Drawing for the job (mm, zero at the part's lowest x, y, z). Coordinates: 2 decimals unless noted, no trailing zeros. Write each loop counter-clockwise with the first axis right and the second up, starting at its lowest first coordinate (ties: lowest second). Pieces come first, ordered by that corner, then holes. Notation, with made-up numbers: M 35,-26 L 59,-26 A29 ccw 59,1 Z; hole C 68,64.5 d9. An arc over 180 degrees is marked long. Use a Markdown table: item, result. Add a question column.
Q1. Wall check: L1, parallel to Y at x = 7, z = 17.78 (3 decimals); L2, parallel to Y at x = 4.25, z = 18.5; L3, parallel to Z at x = 7.5, y = 101.6. Give the ranges that are in metal, low to high. Write a range as from..to.
Q2. Pin check, flat tip, straight feed: pin 1 Ø2 at (y, z) = (25.4, 5.92) entering from +X. Stop position of the tip, or through.
Q3. Slice it at C-C on x = 4. Count the separate pieces of the cut face and the enclosed holes in it, then the cut area to 3 significant figures.
Q4. Slice it at A-A on y = 101.6. Write the cut outline in (x, z) (1 decimal), then the cut area to 3 significant figures.
Q5. Slice it at B-B on y = 63.5. Write the cut outline in (x, z) (1 decimal).
Q6. Slice it at D-D on z = 15.75. Write the cut outline in (x, y) (1 decimal).
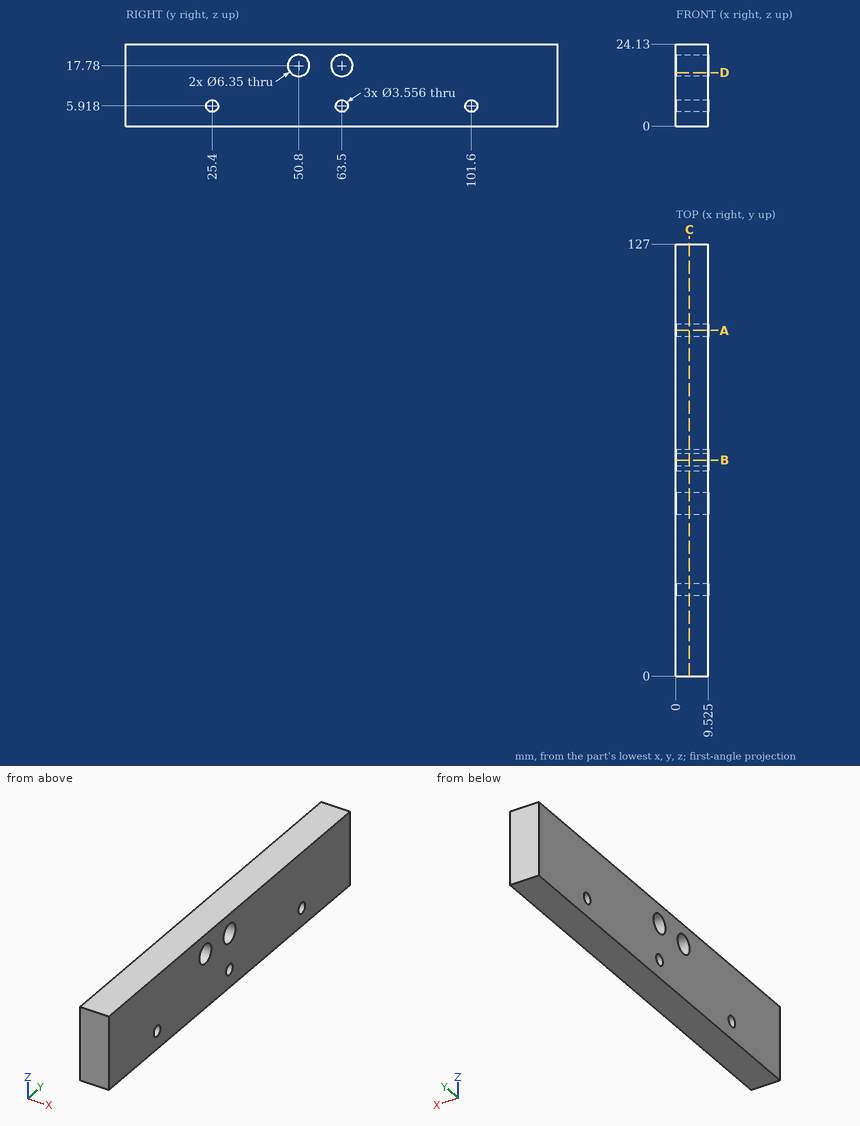
Recorded:
| question | item | result |
|---|---|---|
| 1 | L1 | 0..47.625, 53.975..60.325, 66.675..127 |
| 1 | L2 | 0..47.71, 53.89..60.41, 66.59..127 |
| 1 | L3 | 0..4.14, 7.7..24.13 |
| 2 | pin 1 | through |
| 3 | separate pieces | 1 |
| 3 | enclosed holes | 5 |
| 3 | area | 2,970 mm² |
| 4 | outline | M 0,0 L 9.5,0 L 9.5,4.1 L 0,4.1 Z; M 0,7.7 L 9.5,7.7 L 9.5,24.1 L 0,24.1 Z |
| 4 | area | 196 mm² |
| 5 | outline | M 0,0 L 9.5,0 L 9.5,4.1 L 0,4.1 Z; M 0,7.7 L 9.5,7.7 L 9.5,14.6 L 0,14.6 Z; M 0,21 L 9.5,21 L 9.5,24.1 L 0,24.1 Z |
| 6 | outline | M 0,0 L 9.5,0 L 9.5,48.4 L 0,48.4 Z; M 0,53.2 L 9.5,53.2 L 9.5,61.1 L 0,61.1 Z; M 0,65.9 L 9.5,65.9 L 9.5,127 L 0,127 Z |
